from build123d import *

# Parameters (mm, degrees)
SKETCH1_W           = 21
SKETCH1_H           = 44
BOSS_EXTRUDE1_DEPTH = 2
SKETCH2_R           = 1.6
CUT_EXTRUDE1_DEPTH  = 3
SKETCH3_R           = 4
BOSS_EXTRUDE2_DEPTH = 8


with BuildPart() as part:
    # Sketch1 → Boss-Extrude1 (new body)
    with BuildSketch(Plane.XY):
        with Locations((10.5, 22)):
            Rectangle(SKETCH1_W, SKETCH1_H)
    extrude(amount=BOSS_EXTRUDE1_DEPTH)

    # Sketch2 → Cut-Extrude1 (cut, through all)
    with BuildSketch(Plane.XY.offset(2)):
        with Locations((18.3, 37.1)):
            Circle(SKETCH2_R)
        with Locations((2.7, 6.9)):
            Circle(SKETCH2_R)
    extrude(amount=-CUT_EXTRUDE1_DEPTH, mode=Mode.SUBTRACT)

    # Sketch3 → Boss-Extrude2 (add)
    with BuildSketch(Plane.XY.offset(2)):
        with Locations((10.5, 39.5)):
            Circle(SKETCH3_R)
        with Locations((10.5, 4.5)):
            Circle(SKETCH3_R)
    extrude(amount=BOSS_EXTRUDE2_DEPTH)


solid = part.part
Design review of the part built by this model. Coordinates are the model's own, in mm. A direction names the side the tool comes from. Coordinates: 2 decimals unless noted, no trailing zeros. Order: outer loops, then holes, each group sorted by start corner. A loop starts at its lowest first (then second) coordinate and runs counter-clockwise, first axis right, second up. Notation, with made-up numbers: M 82.5,-19.75 L 101.5,-19.75 A28 cw 101.5,15.25 Z; hole C 62.5,51 d3. An arc over 180 degrees is marked long. Use a Markdown table: item, result.
(1) Add section C-C (z = 4.25). Give the boundary of the cut face in (x, y), then the cut area to 3 significant figures.
Worked answers:
| item | result |
|---|---|
| outline | C 10.5,4.5 d8; C 10.5,39.5 d8 |
| area | 101 mm2 |
(2) Add section A-A (x = 2.7). Give the boundary of the cut face in (y, z), then the cut area to 3 significant figures.
Worked answers:
| item | result |
|---|---|
| outline | M 0,0 L 5.3,0 L 5.3,2 L 0,2 Z; M 8.5,0 L 44,0 L 44,2 L 8.5,2 Z |
| area | 81.6 mm2 |
(3) Add section B-B (y = 37.1). Give the boundary of the cut face in (x, z), then the cut area to 3 significant figures.
Worked answers:
| item | result |
|---|---|
| outline | M 0,0 L 16.7,0 L 16.7,2 L 13.7,2 L 13.7,10 L 7.3,10 L 7.3,2 L 0,2 Z; M 19.9,0 L 21,0 L 21,2 L 19.9,2 Z |
| area | 86.8 mm2 |
(4) For P1, Ø1, axis at x = 8.5, z = 5.5, coming from the +Y side; P2, Ø6, axis at x = 9.5, y = 26.5, coming from the +Z side; P3, Ø1.9, axis at x = 2.7, y = 6.9, coming from the +Z side; P4, Ø1, axis at x = 8.5, z = 8.5, coming from the -Y side, all flat-tipped, find the tip position at first contact; note any pin that passes through.
Worked answers:
| item | result |
|---|---|
| P1 | stops at y = 43.21 |
| P2 | stops at z = 2 |
| P3 | passes through |
| P4 | stops at y = 0.79 |
(5) For faces 4 (the cylindrical face through (9.979, 43.466, 5.944)), 5 (the flat face through (10, 40, 10)), list the 3-axis set-ups (+Z, -Z, +X, -X, +Y, -Y) from which the entire face can be reached by the end or side of a thin tool; tool diameter is ignored.
Worked answers:
| item | result |
|---|---|
| face 4 | +Z |
| face 5 | +Z, +X, -X, +Y, -Y |
(6) Draft analysis for pull direction X (two halves, no side actions). For faces 1 (the flat face through (10, 22, 2)), 2 (the flat face through (21, 22, 1)), 3 (the cylindrical face through (1.1, 6.97, 1.01)), state which applies: released by +X, released by -X, zero draft, split by the parting line, or undercut.
Worked answers:
| item | result |
|---|---|
| face 1 | zero draft |
| face 2 | released by +X |
| face 3 | undercut |
(7) Wall thickness on probe 1 along Y at (x, z) = (18.3, 0.65); probe 2 along Y at (x, z) = (2.7, 0.8); probe 3 along Z at (x, y) = (5.5, 32): over which ranges is each line inside the solid? List them lowest first.
Worked answers:
| item | result |
|---|---|
| probe 1 | y = 0 to 35.5, 38.7 to 44 |
| probe 2 | y = 0 to 5.3, 8.5 to 44 |
| probe 3 | z = 0 to 2 |
(8) Add section D-D (x = 10.5). Give the boundary of the cut face in (y, z), then the cut area to 3 significant figures.
Worked answers:
| item | result |
|---|---|
| outline | M 0,0 L 44,0 L 44,2 L 43.5,2 L 43.5,10 L 35.5,10 L 35.5,2 L 8.5,2 L 8.5,10 L 0.5,10 L 0.5,2 L 0,2 Z |
| area | 216 mm2 |
